Geometry check sheet. Reference: drawing and pictorial views, mm from the part's lowest x, y, z. A direction names the side the tool comes from. Give positions to 0.01 mm unless a question says otherwise; leave off trailing zeros. Write each loop counter-clockwise with the first axis right and the second up, starting at its lowest first coordinate (ties: lowest second). Pieces come first, ordered by that corner, then holes. Notation, with made-up numbers: (22.5, 33.25) - (69.5, 33.25) arc R23 cw to (69.5, 69.25) - close; hole circle Ø2 at (37, 63.5). An arc over 180 degrees is marked (long way). Write item = value, one per line. Start each with the question number.
(1) Depth check by flat-ended pin: pin 1 Ø1 at (x, z) = (19.5, 4.5) entering from +Y; pin 2 Ø2.5 at (x, z) = (10, 3) entering from -Y. Enter the tip coordinate at first touch or a pass-through.
(2) Section check B-B, the plane x = 15.9. Enter the section's corners in (y, z) (3 decimals), plus the area to 3 significant figures.
(3) Access from +Z, -Z, +X, -X, +Y, -Y to the whole of each face (thin tool, end or side, straight path). Record for the marked faces 1, 2 and 3.
(4) Draft check along X on the marked faces 4, 5 and 6. Enter one of: pulls with the +X half, pulls with the -X half, needs draft (parallel to the pull), parting line crosses it, or undercut.
(5) Thickness scan on L1, parallel to X at y = 4.15, z = 4.5; L2, parallel to X at y = 4.3, z = 3.5; L3, parallel to Z at x = 10.25, y = 1. Record the ranges inside material, lowest first.
(6) Section check A-A, the plane y = 4.55. Enter the section's corners in (x, z) (3 decimals).
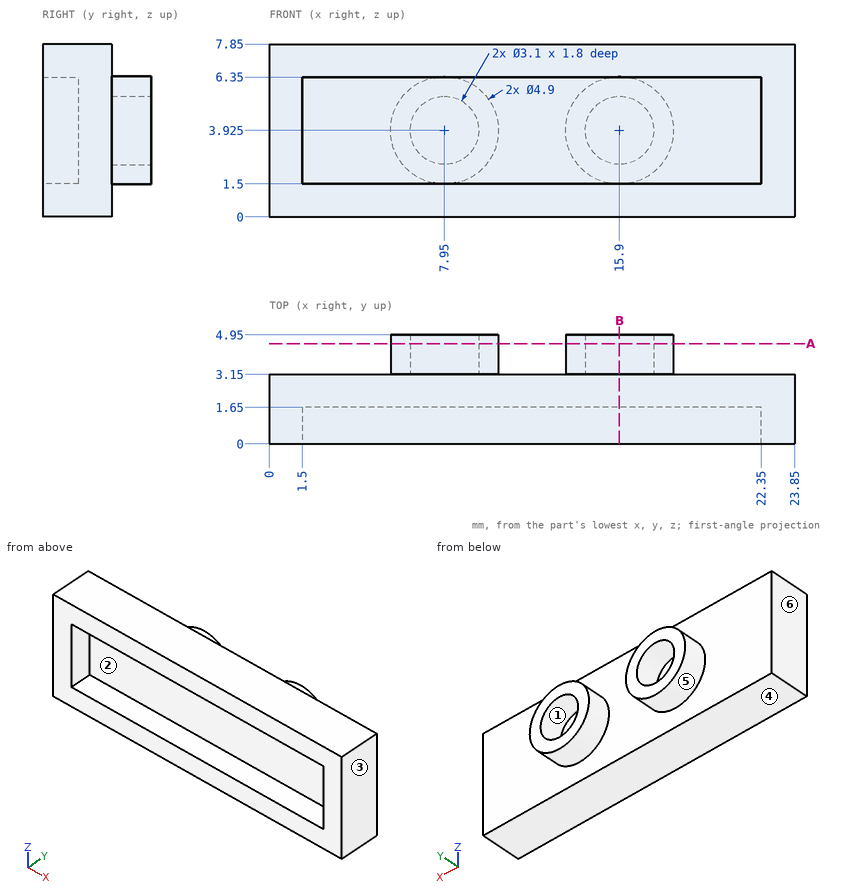
Model answer:
q1.pin_1 = 3.15
q1.pin_2 = 1.65
q2.outline = (0, 0) - (3.15, 0) - (3.15, 1.475) - (4.95, 1.475) - (4.95, 2.375) - (3.15, 2.375) - (3.15, 5.475) - (4.95, 5.475) - (4.95, 6.375) - (3.15, 6.375) - (3.15, 7.85) - (0, 7.85) - (0, 6.35) - (1.65, 6.35) - (1.65, 1.5) - (0, 1.5) - close
q2.area = 20.0 mm²
q3.face_1 = +Y
q3.face_2 = -Y
q3.face_3 = +Z, -Z, +X, +Y, -Y
q4.face_4 = needs draft
q4.face_5 = undercut
q4.face_6 = pulls with the -X half
q5.L1 = 5.57 to 6.51, 9.39 to 10.33, 13.52 to 14.46, 17.34 to 18.28
q5.L2 = 5.54 to 6.46, 9.44 to 10.36, 13.49 to 14.41, 17.39 to 18.31
q5.L3 = 0 to 1.5, 6.35 to 7.85
q6.outline = circle Ø4.9 at (7.95, 3.925); circle Ø4.9 at (15.9, 3.925); hole circle Ø3.1 at (7.95, 3.925); hole circle Ø3.1 at (15.9, 3.925)
